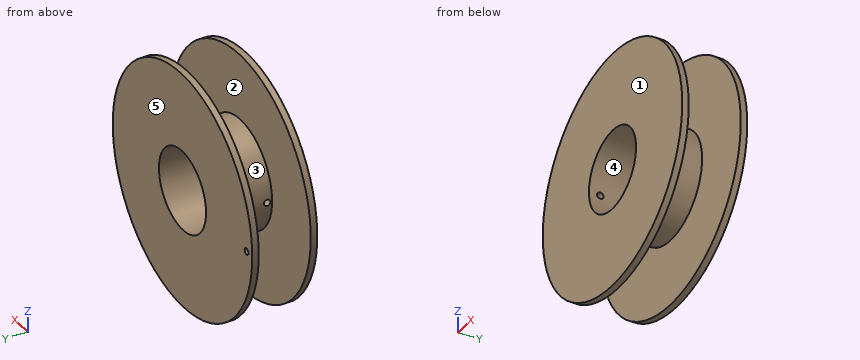
from build123d import *

# Parameters (mm, degrees)
SKETCH_2_R          = 6.75
SKETCH_2_R_2        = 6.25
EXTRUDE_1_DEPTH     = 5
SKETCH_3_R          = 18.5
SKETCH_3_R_2        = 6.75
EXTRUDE_4_DEPTH     = 5
SKETCH_6_R          = 18.5
SKETCH_6_R_2        = 8.25
CUT_EXTRUDE_3_DEPTH = 4
SKETCH_7_R          = 0.5
CUT_EXTRUDE_4_DEPTH = 27.636441204
CUT_EXTRUDE_5_REACH = 30.009
SKETCH_8_R          = 0.5


with BuildPart() as part:
    # 草图2 → 凸台-拉伸1 (new, symmetric)
    with BuildSketch(Plane(origin=(0, 0, 0), x_dir=(1, 0, 0), z_dir=(0, 1, 0))):
        with Locations(Location((0, 0, 0), (0, 0, 270))):
            Circle(SKETCH_2_R)
        with Locations(Location((0, 0, 0), (0, 0, 270))):
            Circle(SKETCH_2_R_2, mode=Mode.SUBTRACT)
    extrude(amount=EXTRUDE_1_DEPTH, both=True)

    # 草图3 → 凸台-拉伸4 (add, symmetric)
    with BuildSketch(Plane(origin=(0, 0, 0), x_dir=(1, 0, 0), z_dir=(0, 1, 0))):
        with Locations(Location((0, 0, 0), (0, 0, 270))):
            Circle(SKETCH_3_R)
        Circle(SKETCH_3_R_2, mode=Mode.SUBTRACT)
    extrude(amount=EXTRUDE_4_DEPTH, both=True)

    # 草图6 → 切除-拉伸3 (cut, symmetric)
    with BuildSketch(Plane(origin=(0, 0, 0), x_dir=(1, 0, 0), z_dir=(0, 1, 0))):
        with Locations(Location((0, 0, 0), (0, 0, 270))):
            Circle(SKETCH_6_R)
        with Locations(Location((0, 0, 0), (0, 0, 270))):
            Circle(SKETCH_6_R_2, mode=Mode.SUBTRACT)
    extrude(amount=CUT_EXTRUDE_3_DEPTH, both=True, mode=Mode.SUBTRACT)

    # 草图7 → 切除-拉伸4 (cut, through all)
    with BuildSketch(Plane(origin=(0, 0, 0), x_dir=(0, 0, -1), z_dir=(1, 0, 0))):
        with Locations((0, -3.25)):
            Circle(SKETCH_7_R)
    extrude(amount=-CUT_EXTRUDE_4_DEPTH, mode=Mode.SUBTRACT)

    # 草图8 → 切除-拉伸5 (cut, up to next)
    with BuildSketch(Plane(origin=(0, 5, 0), x_dir=(1, 0, 0), z_dir=(0, 1, 0)), mode=Mode.PRIVATE) as cut_extrude_5_sk1:
        with Locations(Location((-17, 0, 0), (0, 0, 270))):
            Circle(SKETCH_8_R)
    cut_extrude_5_tool1 = extrude(cut_extrude_5_sk1.sketch, amount=-CUT_EXTRUDE_5_REACH, mode=Mode.PRIVATE) & part.part
    add(cut_extrude_5_tool1.solids().sort_by_distance((-17, 5, 0))[0], mode=Mode.SUBTRACT)


solid = part.part
Geometry: final body of the model. Coordinates: model frame, mm. Face numbers are marked on the shaded views. A direction names the side the tool comes from. Coordinates: 2 decimals unless noted, no trailing zeros. Order: outer loops, then holes, each group sorted by start corner. A loop starts at its lowest first (then second) coordinate and runs counter-clockwise, first axis right, second up.
(1) Material intervals for probe 1 along Y at (x, z) = (-10.5, 1); probe 2 along X at (y, z) = (-2, 0); probe 3 along Y at (x, z) = (-7.2, 0), sorted ascending.
(2) Draft query along X for the marked faces 3, 4 and 5. Return one class per face: pulls with the +X half, pulls with the -X half, needs draft (parallel to the pull), parting line crosses it, or undercut.
(3) Section query B-B (z = 0). Return the cut outline in (x, y).
(4) Section query D-D (x = -17). Return the cut outline in (y, z).
(5) First-contact query: pin 1 (2 mm diameter, centred on y = 1, z = -6, fed in from +X); pin 2 (10 mm diameter, centred on x = 2, z = 4, fed in from -Y); pin 3 (4 mm diameter, centred on y = -2.5, z = 1, fed in from +X). Flat tips, straight axial feed; report the tip coordinate or a pass-through.
(6) Section query A-A (x = 0). Return the cut outline in (y, z).
(7) Section query C-C (z = -16). Return the cut outline in (x, y).
(8) Access query for the marked faces 1 and 2. Directions: +Z, -Z, +X, -X, +Y, -Y. A direction counts if a zero-diameter tool reaches every point of the face in a straight line with its end or side. Return the directions, or none.
Solution:
1. probe 1: y = -5 to -4, 4 to 5
1. probe 2: x = -8.25 to -6.25, 6.25 to 8.25
1. probe 3: y = -5 to -3.75, -2.75 to 5
2. face 3: parting line crosses it
2. face 4: undercut
2. face 5: needs draft
3. outline: (-18.5, -5) - (-6.25, -5) - (-6.25, -3.75) - (-8.25, -3.75) - (-8.25, -4) - (-18.5, -4) - close; (-18.5, 4) - (-17.5, 4) - (-17.5, 5) - (-18.5, 5) - close; (-16.5, 4) - (-8.25, 4) - (-8.25, -2.75) - (-6.25, -2.75) - (-6.25, 5) - (-16.5, 5) - close; (6.25, -5) - (18.5, -5) - (18.5, -4) - (8.25, -4) - (8.25, 4) - (18.5, 4) - (18.5, 5) - (6.25, 5) - close
4. outline: (-5, -7.3) - (-4, -7.3) - (-4, 7.3) - (-5, 7.3) - close; (4, -7.3) - (5, -7.3) - (5, -0.5) - (4, -0.5) - close; (4, 0.5) - (5, 0.5) - (5, 7.3) - (4, 7.3) - close
5. pin 1: stops at x = 6.56
5. pin 2: stops at y = -5
5. pin 3: stops at x = 18.5
6. outline: (-5, -18.5) - (-4, -18.5) - (-4, -8.25) - (4, -8.25) - (4, -18.5) - (5, -18.5) - (5, -6.25) - (-5, -6.25) - close; (-5, 6.25) - (5, 6.25) - (5, 18.5) - (4, 18.5) - (4, 8.25) - (-4, 8.25) - (-4, 18.5) - (-5, 18.5) - close
7. outline: (-9.29, -5) - (9.29, -5) - (9.29, -4) - (-9.29, -4) - close; (-9.29, 4) - (9.29, 4) - (9.29, 5) - (-9.29, 5) - close
8. face 1: +Z, -Z, +X, -X, -Y
8. face 2: none
